Autodesk Inventor part; units mm, degrees
ref_plane "YZ Plane" through (0, 0, 0) normal (1, 0, 0) x (0, 1, 0)
ref_plane "XZ Plane" through (0, 0, 0) normal (0, 1, 0) x (-1, 0, 0)
ref_plane "XY Plane" through (0, 0, 0) normal (0, 0, 1) x (1, 0, 0)
sketch "スケッチ1" plane through (0, 0, 0) normal (0, 1, 0) x (-1, 0, 0)
  line L0 (0, 99) -> (20, 99)
  line L1 (20, 99) -> (20, -99)
  line L2 (20, -99) -> (0, -99)
  line L3 (0, -99) -> (0, 99)
  line L4 (20, -99) -> (20, -109)
  line L5 (20, -109) -> (9, -109)
  line L6 (9, -109) -> (11, -99)
  line L7 (10.5, 99) -> (8.5, 88.5)
  line L8 (8.5, 88.5) -> (20, 88.5)
  point P0 (0, 0)
  point P1 (0, 0)
  point P2 (10, -99)
  point P3 (10, 99)
  dimension "d0" = 198
  dimension "d1" = 20
  dimension "d4" = 10
  dimension "d5" = 1
  dimension "d6" = 1
  dimension "d7" = 10.5
  dimension "d8" = 1.5
  dimension "d9" = 0.5
extrude "押し出し1" add sketch "スケッチ1" along normal blind 5.5 contours L0 L7 L8 L1 L2 L3 | L2 L4 L5 L6
sketch "スケッチ2" plane through (0, 5.5, 0) normal (0, 1, 0) x (1, 0, 0)
  line L0 (-20, 109) -> (-20, -88.5)
  line L1 (-20, -1.5) -> (-17, -1.5)
  line L2 (-17, -1.5) -> (-17, 1.5)
  line L3 (-17, 1.5) -> (-20, 1.5)
  line L4 (-20, 1.5) -> (-20, -1.5)
  line L5 (0, -99) -> (0, 99)
  line L6 (0, -1.5) -> (-3, -1.5)
  line L7 (-3, -1.5) -> (-3, 1.5)
  line L8 (-3, 1.5) -> (0, 1.5)
  line L9 (0, 1.5) -> (0, -1.5)
  point P0 (0, 0)
  point P1 (-17, 0)
  point P2 (0, 0)
  point P3 (0, 1.5)
  dimension "d10" = 3
  dimension "d11" = 3
extrude "押し出し2" cut sketch "スケッチ2" against normal through all
pattern_linear "矩形状パターン1" count 3 spacing 40 along (0, 0, -1) count 3 spacing 40 along (0, 0, 1) of "押し出し2"
properties part number "front" material "木材 (カエデ材)"
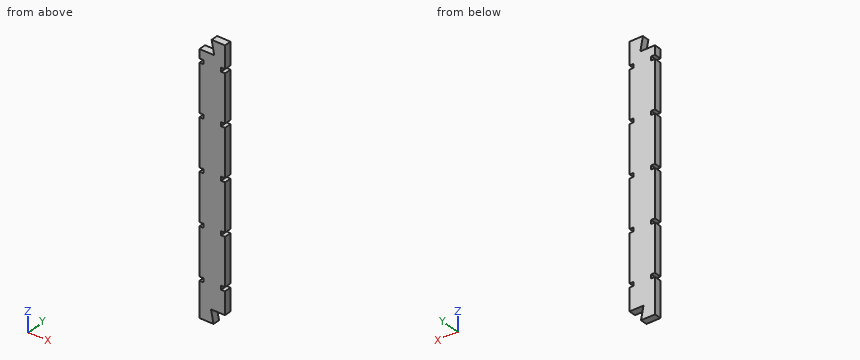
Part model, mm, in its own coordinate system. Round coordinates to 2 decimals unless told otherwise and drop trailing zeros. Write each loop counter-clockwise with the first axis right and the second up, starting at its lowest first coordinate (ties: lowest second). Pieces come first, ordered by that corner, then holes. Notation, with made-up numbers: M 36.5,-32 L 51.5,-32 A36 cw 51.5,2 Z; hole C 18.5,-2.75 d6. An arc over 180 degrees is marked long. One line per question, with ' | ' between items.
(1) Saw through at A-A on x = -5.25. Write the cut outline in (y, z).
Answer key:
outline: M 0,-99 L 5.5,-99 L 5.5,99 L 0,99 Z
(2) Probe line 1 along Z through (x, y) = (-18.5, 3); line 2 along Z through (x, y) = (-14, 3.1); line 3 along Z through (x, y) = (-5, 1.6). List the from-to ranges inside material, lowest first.
Answer key:
line 1: z = -109 to -81.5, -78.5 to -41.5, -38.5 to -1.5, 1.5 to 38.5, 41.5 to 78.5, 81.5 to 88.5 | line 2: z = -109 to 88.5 | line 3: z = -99 to 99
(3) Pin check, flat tips, straight feed: pin 1 (1.5 mm diameter, centred on x = -1, y = 1.5, fed in from -Z); pin 2 (0.9 mm diameter, centred on x = -19, y = 2.5, fed in from +Z); pin 3 (0.9 mm diameter, centred on y = 2.5, z = 80, fed in from -X). Stop position of each tip, or through.
Answer key:
pin 1: stops at z = -99 | pin 2: stops at z = 88.5 | pin 3: stops at x = -17
